Geometry: final body of the model. Coordinates: model frame, mm. A direction names the side the tool comes from. Coordinates: 2 decimals unless noted, no trailing zeros. Write each loop counter-clockwise with the first axis right and the second up, starting at its lowest first coordinate (ties: lowest second). Pieces come first, ordered by that corner, then holes.
from build123d import *

# Parameters (mm, degrees)
SKETCH_2_R      = 2.25
EXTRUDE_1_DEPTH = 5


with BuildPart() as part:
    # 草图2 → 凸台-拉伸1 (new body)
    with BuildSketch(Plane(origin=(0, 0, 0), x_dir=(1, 0, 0), z_dir=(0, 1, 0))):
        Polygon((-11.75, 45), (-52.25, 45), (-52.25, -45), (52.25, -45), (52.25, 45), (11.75, 45), (11.75, 21), (-11.75, 21), align=None)
        with Locations(Location((-48, -40.75, 0), (0, 0, 270))):
            Circle(SKETCH_2_R, mode=Mode.SUBTRACT)
        with Locations(Location((-40, -40.75, 0), (0, 0, 270))):
            Circle(SKETCH_2_R, mode=Mode.SUBTRACT)
        with Locations(Location((-32, -40.75, 0), (0, 0, 270))):
            Circle(SKETCH_2_R, mode=Mode.SUBTRACT)
        with Locations(Location((-24, -40.75, 0), (0, 0, 270))):
            Circle(SKETCH_2_R, mode=Mode.SUBTRACT)
        with Locations(Location((-16, -40.75, 0), (0, 0, 270))):
            Circle(SKETCH_2_R, mode=Mode.SUBTRACT)
        with Locations(Location((16, -40.75, 0), (0, 0, 270))):
            Circle(SKETCH_2_R, mode=Mode.SUBTRACT)
        with Locations(Location((24, -40.75, 0), (0, 0, 270))):
            Circle(SKETCH_2_R, mode=Mode.SUBTRACT)
        with Locations(Location((32, -40.75, 0), (0, 0, 270))):
            Circle(SKETCH_2_R, mode=Mode.SUBTRACT)
        with Locations(Location((40, -40.75, 0), (0, 0, 270))):
            Circle(SKETCH_2_R, mode=Mode.SUBTRACT)
        with Locations(Location((48, -40.75, 0), (0, 0, 270))):
            Circle(SKETCH_2_R, mode=Mode.SUBTRACT)
        with Locations(Location((-8, 16.75, 0), (0, 0, 270))):
            Circle(SKETCH_2_R, mode=Mode.SUBTRACT)
        with Locations(Location((-48, 40.75, 0), (0, 0, 270))):
            Circle(SKETCH_2_R, mode=Mode.SUBTRACT)
        with Locations(Location((-40, 40.75, 0), (0, 0, 270))):
            Circle(SKETCH_2_R, mode=Mode.SUBTRACT)
        with Locations(Location((-32, 40.75, 0), (0, 0, 270))):
            Circle(SKETCH_2_R, mode=Mode.SUBTRACT)
        with Locations(Location((-24, 40.75, 0), (0, 0, 270))):
            Circle(SKETCH_2_R, mode=Mode.SUBTRACT)
        with Locations(Location((-16, 40.75, 0), (0, 0, 270))):
            Circle(SKETCH_2_R, mode=Mode.SUBTRACT)
        with Locations(Location((0, 16.75, 0), (0, 0, 270))):
            Circle(SKETCH_2_R, mode=Mode.SUBTRACT)
        with Locations(Location((8, 16.75, 0), (0, 0, 270))):
            Circle(SKETCH_2_R, mode=Mode.SUBTRACT)
        with Locations(Location((16, 40.75, 0), (0, 0, 270))):
            Circle(SKETCH_2_R, mode=Mode.SUBTRACT)
        with Locations(Location((24, 40.75, 0), (0, 0, 270))):
            Circle(SKETCH_2_R, mode=Mode.SUBTRACT)
        with Locations(Location((32, 40.75, 0), (0, 0, 270))):
            Circle(SKETCH_2_R, mode=Mode.SUBTRACT)
        with Locations(Location((40, 40.75, 0), (0, 0, 270))):
            Circle(SKETCH_2_R, mode=Mode.SUBTRACT)
        with Locations(Location((48, 40.75, 0), (0, 0, 270))):
            Circle(SKETCH_2_R, mode=Mode.SUBTRACT)
    extrude(amount=EXTRUDE_1_DEPTH)


solid = part.part
Item 1: Material intervals for probe 1 along Z at (x, y) = (26, 0.9); probe 2 along X at (y, z) = (2.2, -16.75); probe 3 along Z at (x, y) = (32.5, 3.3), sorted ascending.
Derived:
probe 1: z = -45 to -41.78, -39.72 to 39.72, 41.78 to 45
probe 2: x = -52.25 to -10.25, -5.75 to -2.25, 2.25 to 5.75, 10.25 to 52.25
probe 3: z = -45 to -42.94, -38.56 to 38.56, 42.94 to 45
Item 2: Set-up query: faces 4 (the flat face through (0, 2, -21)), 5 (the cylindrical face through (-31.901, 2.465, 38.502)). Return all of +Z, -Z, +X, -X, +Y, -Y with unobstructed straight access to the full face (end or side cutting, diameter ignored); none if empty.
Derived:
face 4: -Z, +Y, -Y
face 5: +Y, -Y
Item 3: Section D-D, the plane x = -16. Output: boundary loops of the cut face in (y, z), plus the area to 3 significant figures.
Derived:
outline: (0, -45) - (5, -45) - (5, -43) - (0, -43) - close; (0, -38.5) - (5, -38.5) - (5, 38.5) - (0, 38.5) - close; (0, 43) - (5, 43) - (5, 45) - (0, 45) - close
area: 405 mm2
Item 4: Section C-C, the plane z = -16.75. Output: boundary loops of the cut face in (x, y), plus the area to 3 significant figures.
Derived:
outline: (-52.25, 0) - (-10.25, 0) - (-10.25, 5) - (-52.25, 5) - close; (-5.75, 0) - (-2.25, 0) - (-2.25, 5) - (-5.75, 5) - close; (2.25, 0) - (5.75, 0) - (5.75, 5) - (2.25, 5) - close; (10.25, 0) - (52.25, 0) - (52.25, 5) - (10.25, 5) - close
area: 455 mm2
Item 5: Pull-direction query (Z, two-part tool) for faces 1 (the flat face through (32, 2, -45)), 2 (the cylindrical face through (50.23, 2.46, 40.46)), 3 (the flat face through (-11.75, 2, -33)); classes: released by +Z, released by -Z, zero draft, split by the parting line, or undercut.
Derived:
face 1: released by -Z
face 2: undercut
face 3: zero draft
Item 6: Section B-B, the plane y = 1.2. State how many separate pieces and enclosed holes the cut face has, plus the area to 3 significant figures.
Derived:
separate pieces: 1
enclosed holes: 23
area: 8,480 mm2
Item 7: Section A-A, the plane x = 8. Output: boundary loops of the cut face in (y, z).
Derived:
outline: (0, -21) - (5, -21) - (5, -19) - (0, -19) - close; (0, -14.5) - (5, -14.5) - (5, 45) - (0, 45) - close
